Check sheet for the modelled part. Datum: model origin and axes. Units: mm. A direction names the side the tool comes from. Give positions to 0.01 mm unless a question says otherwise; leave off trailing zeros. Loops run counter-clockwise (first coordinate to the right, second up) from the corner with the lowest first, then second, coordinate; pieces in that order, holes last. Notation, with made-up numbers: (43.25, -37) - (66.25, -37) arc R20 ccw to (66.25, -10) - close; hole circle Ø8 at (34, -2). An arc over 180 degrees is marked (long way). Use one line per item in the form item = value.
from build123d import *

# Parameters (mm, degrees)
F0_W     = 520
F0_H     = 27
F1_DEPTH = 7
F2_W     = 158
F2_H     = 96.179498
F2_W_2   = 50
F3_DEPTH = 25


with BuildPart() as f1:
    # F0 (on Top) → F1 (new body)
    with BuildSketch(Plane.XY):
        Rectangle(F0_W, F0_H)
        with BuildLine():
            ThreePointArc((-92.5, 8), (-86.843146, 5.656854), (-84.5, 0))
            ThreePointArc((-84.5, 0), (-86.843146, -5.656854), (-92.5, -8))
            Line((-92.5, -8), (-108.5, -8))
            ThreePointArc((-108.5, -8), (-116.5, 0), (-108.5, 8))
            Line((-108.5, 8), (-92.5, 8))
        make_face(mode=Mode.SUBTRACT)
        with BuildLine():
            ThreePointArc((-19.5, 8), (-13.843146, 5.656854), (-11.5, 0))
            ThreePointArc((-11.5, 0), (-13.843146, -5.656854), (-19.5, -8))
            Line((-19.5, -8), (-35.5, -8))
            ThreePointArc((-35.5, -8), (-43.5, 0), (-35.5, 8))
            Line((-35.5, 8), (-19.5, 8))
        make_face(mode=Mode.SUBTRACT)
        with BuildLine():
            ThreePointArc((53.5, 8), (59.156854, 5.656854), (61.5, 0))
            ThreePointArc((61.5, 0), (59.156854, -5.656854), (53.5, -8))
            Line((53.5, -8), (37.5, -8))
            ThreePointArc((37.5, -8), (29.5, 0), (37.5, 8))
            Line((37.5, 8), (53.5, 8))
        make_face(mode=Mode.SUBTRACT)
        with BuildLine():
            ThreePointArc((126.5, 8), (132.156854, 5.656854), (134.5, 0))
            ThreePointArc((134.5, 0), (132.156854, -5.656854), (126.5, -8))
            Line((126.5, -8), (110.5, -8))
            ThreePointArc((110.5, -8), (102.5, 0), (110.5, 8))
            Line((110.5, 8), (126.5, 8))
        make_face(mode=Mode.SUBTRACT)
        with BuildLine():
            ThreePointArc((199.5, 8), (205.156854, 5.656854), (207.5, 0))
            ThreePointArc((207.5, 0), (205.156854, -5.656854), (199.5, -8))
            Line((199.5, -8), (183.5, -8))
            ThreePointArc((183.5, -8), (175.5, 0), (183.5, 8))
            Line((183.5, 8), (199.5, 8))
        make_face(mode=Mode.SUBTRACT)
    extrude(amount=F1_DEPTH)

    # F2 (on face) → F3 (cut)
    with BuildSketch(Plane.XY.offset(7)):
        with Locations((23, -3.07426)):
            Rectangle(F2_W, F2_H)
        with Locations((-135, -3.07426)):
            Rectangle(F2_W, F2_H)
        with Locations((-239, -3.07426)):
            Rectangle(F2_W_2, F2_H)
    extrude(amount=-F3_DEPTH, mode=Mode.SUBTRACT)


solid = f1.part
Item 1: Section check C-C on z = 2.25. Record the boundary of the cut face in (x, y).
Answer block:
outline = (102, -13.5) - (260, -13.5) - (260, 13.5) - (102, 13.5) - close; hole (110.5, -8) - (126.5, -8) arc R8 ccw to (134.5, 0) arc R8 ccw to (126.5, 8) - (110.5, 8) arc R8 ccw to start; hole (183.5, -8) - (199.5, -8) arc R8 ccw to (207.5, 0) arc R8 ccw to (199.5, 8) - (183.5, 8) arc R8 ccw to start
Item 2: Section check B-B on y = -5. Record the boundary of the cut face in (x, z) (3 decimals).
Answer block:
outline = (102, 0) - (104.255, 0) - (104.255, 7) - (102, 7) - close; (132.745, 0) - (177.255, 0) - (177.255, 7) - (132.745, 7) - close; (205.745, 0) - (260, 0) - (260, 7) - (205.745, 7) - close
Item 3: Gauge pin test, flat end, axial feed: P1, Ø4, axis at x = 211.5, y = -3.5, coming from the -Z side. Record the tip position at first contact, or that the pin passes through.
Answer block:
P1 = 0
Item 4: Access from +Z, -Z, +X, -X, +Y, -Y to the whole of each face (thin tool, end or side, straight path). Record for faces 1 (the face through (180, 9, 0)), 2 (the face through (191, 8, 3)).
Answer block:
face_1 = -Z, +X, -X, +Y, -Y
face_2 = +Z, -Z
Item 5: Mould release check, pull along X, two halves, no side actions. Record for faces 3 (the face through (180, 9, 7)), 4 (the face through (192, -8, 3)), 5 (the face through (102, 0, 4)): released by +X, released by -X, zero draft, split by the parting line, or undercut.
Answer block:
face_3 = zero draft
face_4 = undercut
face_5 = released by -X
Item 6: Thickness scan on L1, parallel to X at y = 0.5, z = 6; L2, parallel to X at y = 2, z = 1.5; L3, parallel to Y at x = 112.5, z = 1.25. Record the ranges inside material, lowest first.
Answer block:
L1 = 102 to 102.52, 134.48 to 175.52, 207.48 to 260
L2 = 102 to 102.75, 134.25 to 175.75, 207.25 to 260
L3 = -13.5 to -8, 8 to 13.5
Item 7: Section check A-A on x = 194. Record the boundary of the cut face in (y, z), then the cut area to 3 significant figures.
Answer block:
outline = (-13.5, 0) - (-8, 0) - (-8, 7) - (-13.5, 7) - close; (8, 0) - (13.5, 0) - (13.5, 7) - (8, 7) - close
area = 77.0 mm2
